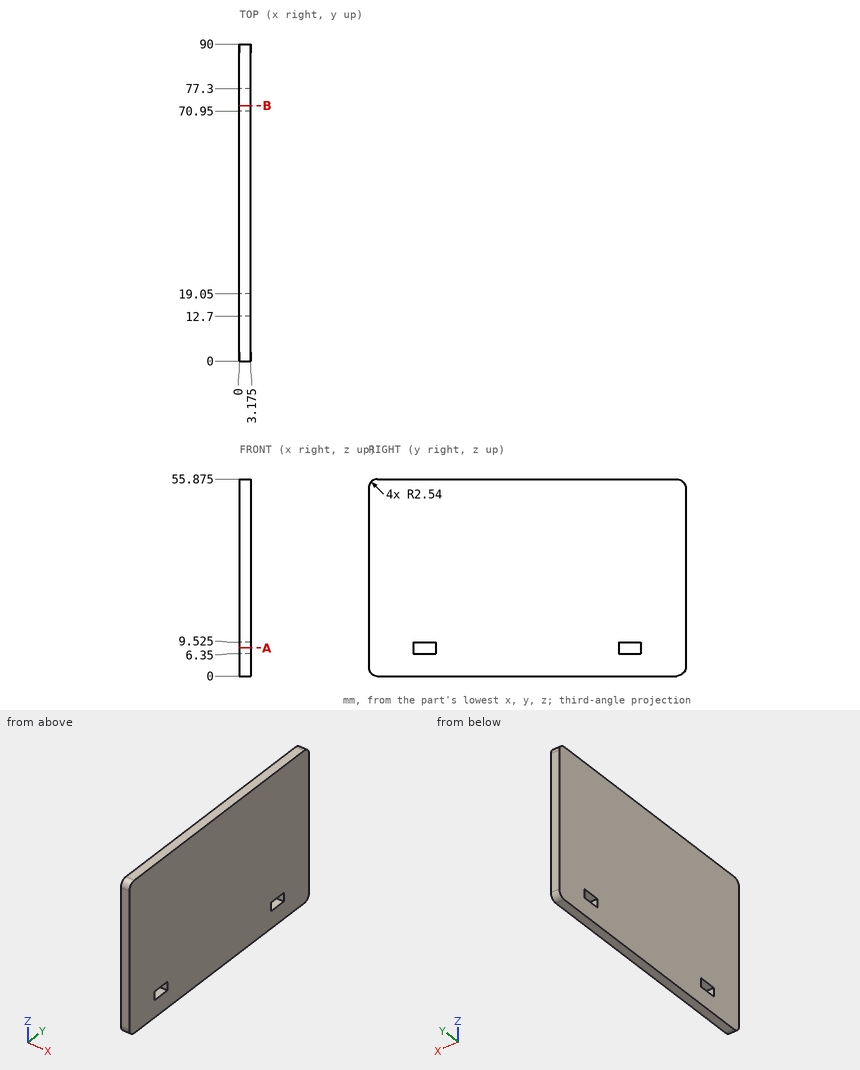
The figure shows three views and two pictorial views of one solid part (mm, origin at its lowest corner). Answer the questions. Give positions to 0.01 mm unless a question says otherwise; leave off trailing zeros. Write each loop counter-clockwise with the first axis right and the second up, starting at its lowest first coordinate (ties: lowest second). Pieces come first, ordered by that corner, then holes. Notation, with made-up numbers: (-33.75, 63.5) - (-0.75, 63.5) arc R18 ccw to (-0.75, 74.5) - close; hole circle Ø11 at (45.25, 22.25). An arc over 180 degrees is marked (long way). Use one line per item in the form item = value.
1. This flat-tipped pin is pushed along its axis until it touches: pin 1 Ø3 at (y, z) = (67.5, 34.5) entering from -X. Where does it stop, or does it pass through?
Filled in:
pin_1 = 0
2. A cutting plane is placed at B-B (y = 72.5). Write down the section's boundary in (x, z) (3 decimals), and give its area (3 significant figures).
Filled in:
outline = (0, 0) - (3.175, 0) - (3.175, 6.35) - (0, 6.35) - close; (0, 9.525) - (3.175, 9.525) - (3.175, 55.875) - (0, 55.875) - close
area = 167 mm^2
3. A cutting plane is placed at A-A (z = 8). Write down the section's boundary in (x, y) (3 decimals), and give its area (3 significant figures).
Filled in:
outline = (0, 0) - (3.175, 0) - (3.175, 12.7) - (0, 12.7) - close; (0, 19.05) - (3.175, 19.05) - (3.175, 70.95) - (0, 70.95) - close; (0, 77.3) - (3.175, 77.3) - (3.175, 90) - (0, 90) - close
area = 245 mm^2
4. Consider L1, parallel to Z at x = 1.9, y = 72.5 (3 decimals). Determine where the line is inside the solid, lowest interval first.
Filled in:
L1 = 0 to 6.35, 9.525 to 55.875
